Part model, mm, in its own coordinate system. A direction names the side the tool comes from. Round coordinates to 2 decimals unless told otherwise and drop trailing zeros. Loops run counter-clockwise (first coordinate to the right, second up) from the corner with the lowest first, then second, coordinate; pieces in that order, holes last. Notation, with made-up numbers: M 69,3.25 L 74,3.25 A22 ccw 74,22.25 Z; hole C 78.5,36 d5. An arc over 180 degrees is marked long. Write each question's results on one line, items separated by ' | '.
Autodesk Inventor part; units mm, degrees
ref_plane "YZ Plane" through (0, 0, 0) normal (1, 0, 0) x (0, 1, 0)
ref_plane "XZ Plane" through (0, 0, 0) normal (0, 1, 0) x (-1, 0, 0)
ref_plane "XY Plane" through (0, 0, 0) normal (0, 0, 1) x (1, 0, 0)
sketch "Sketch1" plane through (0, 0, 0) normal (0, 1, 0) x (-1, 0, 0)
  line L0 (0, 25.4) -> (25.4, 25.4)
  line L1 (25.4, 25.4) -> (25.4, 0)
  line L2 (25.4, 0) -> (0, 0)
  line L3 (0, 0) -> (0, 25.4)
  line L4 (22.225, 22.225) -> (3.175, 22.225)
  line L5 (3.175, 22.225) -> (3.175, 3.175)
  line L6 (3.175, 3.175) -> (22.225, 3.175)
  line L7 (22.225, 3.175) -> (22.225, 22.225)
  dimension "d0" = 25.4
  dimension "d1" = 25.4
  dimension "d2" = 3.175
extrude "Extrusion1" add sketch "Sketch1" along normal blind 609.6
sketch "Sketch2" plane through (-25.4, 0, 25.4) normal (0, 0, 1) x (1, 0, 0)
  circle A0 centre (12.7, 491.5841) radius 3.302
  circle A1 centre (12.7, 452.2611) radius 3.302
  circle A2 centre (12.7, 412.9381) radius 3.302
  circle A3 centre (12.7, 373.6152) radius 3.302
  circle A4 centre (12.7, 334.2922) radius 3.302
  circle A5 centre (12.7, 294.9693) radius 3.302
  circle A6 centre (12.7, 255.6463) radius 3.302
  circle A7 centre (12.7, 216.3233) radius 3.302
  circle A8 centre (12.7, 177.0004) radius 3.302
  circle A9 centre (12.7, 137.6774) radius 3.302
  circle A10 centre (12.7, 98.3544) radius 3.302
  circle A11 centre (12.7, 118.0159) radius 3.302
  circle A12 centre (12.7, 157.3389) radius 3.302
  circle A13 centre (12.7, 196.6619) radius 3.302
  circle A14 centre (12.7, 235.9848) radius 3.302
  circle A15 centre (12.7, 275.3078) radius 3.302
  circle A16 centre (12.7, 314.6307) radius 3.302
  circle A17 centre (12.7, 353.9537) radius 3.302
  circle A18 centre (12.7, 393.2767) radius 3.302
  circle A19 centre (12.7, 432.5996) radius 3.302
  circle A20 centre (12.7, 471.9226) radius 3.302
  circle A21 centre (12.7, 511.2456) radius 3.302
  line L0 (0, 25.4) -> (25.4, 25.4)
  line L1 (0, 25.4) -> (0, 584.2)
  line L2 (25.4, 584.2) -> (0, 584.2)
  line L3 (25.4, 25.4) -> (25.4, 584.2)
extrude "Extrusion2" [suppressed]
sketch "Sketch3" plane through (-25.4, 0, 0) normal (-1, 0, 0) x (0, 0, 1)
  line L0 (25.4, 0) -> (25.4, 609.6)
  line L1 (0, 0) -> (0, 609.6)
  line L2 (0, 511.2456) -> (25.4, 511.2456) construction
  line L3 (0, 373.6152) -> (25.4, 373.6152) construction
  line L4 (0, 235.9848) -> (25.4, 235.9848) construction
  line L5 (0, 98.3544) -> (25.4, 98.3544) construction
  line L6 (12.7, 523.9456) -> (12.7, 479.4956) construction
  line L7 (12.7, 403.7777) -> (12.7, 343.4527) construction
  line L8 (12.7, 258.2098) -> (12.7, 213.7598) construction
  line L9 (12.7, 130.1044) -> (12.7, 85.6544) construction
  circle A0 centre (12.7, 523.9456) radius 3.302
  circle A1 centre (12.7, 479.4956) radius 3.302
  circle A2 centre (12.7, 403.7777) radius 3.302
  circle A3 centre (12.7, 343.4527) radius 3.302
  circle A4 centre (12.7, 258.2098) radius 3.302
  circle A5 centre (12.7, 213.7598) radius 3.302
  circle A6 centre (12.7, 130.1044) radius 3.302
  circle A7 centre (12.7, 85.6544) radius 3.302
  line L10 (0, 304.8) -> (25.4, 304.8) construction
  line L11 (12.7, 334.9625) -> (12.7, 274.6375) construction
  circle A8 centre (12.7, 334.9625) radius 3.302
  circle A9 centre (12.7, 274.6375) radius 3.302
  line L12 (0, 609.6) -> (25.4, 609.6)
  line L13 (0, 107.8794) -> (25.4, 107.8794) construction
  line L14 (25.4, 0) -> (0, 0)
  circle A10 centre (12.7, 596.9) radius 3.302
  circle A11 centre (12.7, 574.675) radius 3.302
  circle A12 centre (12.7, 558.8) radius 3.302
  line L15 (0, 501.7206) -> (25.4, 501.7206) construction
  circle A13 centre (12.7, 12.7) radius 3.302
  circle A14 centre (12.7, 34.925) radius 3.302
  circle A15 centre (12.7, 50.8) radius 3.302
  point P0 (12.7, 235.9848)
  point P1 (12.7, 373.6152)
  point P2 (12.7, 304.8)
  point P3 (12.7, 107.8794)
  point P4 (12.7, 501.7206)
  dimension "d7" = 44.45
  dimension "d8" = 60.325
  dimension "d9" = 44.45
  dimension "d10" = 44.45
  dimension "d11" = 6.604
  dimension "d12" = 6.604
  dimension "d13" = 6.604
  dimension "d14" = 6.604
  dimension "d15" = 6.604
  dimension "d16" = 6.604
  dimension "d17" = 6.604
  dimension "d18" = 6.604
  dimension "d21" = 60.325
  dimension "d22" = 6.604
  dimension "d23" = 6.604
  dimension "d27" = 9.525
  dimension "d28" = 9.525
  dimension "d29" = 98.3544
  dimension "d30" = 235.9848
  dimension "d31" = 235.9848
  dimension "d32" = 98.3544
extrude "Extrusion3" cut sketch "Sketch3" against normal blind 25.4 contours A0 | A1 | A6 | A7 | A8 | A9 | A10 | A11 | A12 | A13 | A14 | A15
sketch "Sketch4" plane through (0, 0, 25.4) normal (1, 0, 0) x (0, 0, -1)
  line L0 (25.4, 0) -> (25.4, 609.6)
  line L1 (0, 0) -> (0, 609.6)
  line L2 (0, 304.8) -> (25.4, 304.8) construction
  line L3 (12.7, 349.25) -> (12.7, 260.35) construction
  circle A0 centre (12.7, 349.25) radius 3.302
  circle A1 centre (12.7, 260.35) radius 3.302
  circle A2 centre (12.7, 368.3) radius 3.302
  circle A3 centre (12.7, 387.35) radius 3.302
  circle A4 centre (12.7, 406.4) radius 3.302
  circle A5 centre (12.7, 425.45) radius 3.302
  circle A6 centre (12.7, 444.5) radius 3.302
  circle A7 centre (12.7, 241.3) radius 3.302
  circle A8 centre (12.7, 222.25) radius 3.302
  circle A9 centre (12.7, 203.2) radius 3.302
  circle A10 centre (12.7, 184.15) radius 3.302
  circle A11 centre (12.7, 165.1) radius 3.302
  point P0 (12.7, 304.8)
  dimension "d33" = 88.9
  dimension "d34" = 6.604
  dimension "d37" = 19.05
  dimension "d44" = 19.05
extrude "Extrusion4" cut sketch "Sketch4" against normal blind 25.4 contours A2 | A3 | A4 | A5 | A6 | A7 | A8 | A9 | A10 | A11
equation "\"d9\" = d7"
equation "\"d10\" = d7"
equation "\"d12\" = d11"
equation "\"d13\" = d11"
equation "\"d14\" = d11"
equation "\"d15\" = d11"
equation "\"d16\" = d11"
equation "\"d17\" = d11"
equation "\"d18\" = d11"
equation "\"d21\" = d8"
equation "\"d22\" = d11"
equation "\"d23\" = d11"
equation "\"d27\" = d28"
properties part number "Chassis V1.500 Part1" material "Aluminum 6061"
Item 1: Drop a flat-ended pin along its axis: P1, Ø4, axis at y = 425.45, z = 12.7, coming from the +X side. Give the stop position or say it passes through.
Filled sheet:
P1: through
Item 2: Two-plate mould, pull along Z, no slides. Class faces 1 (the flat face through (-13, 301, 0)), 2 (the flat face through (-24, 0, 13)), 3 (the flat face through (-13, 301, 3.175)): +Z half, -Z half, draft (parallel to the pull), parting line (faces both ways), or undercut.
Filled sheet:
face 1: -Z half | face 2: draft | face 3: undercut
Item 3: Band-saw the part on B-B on y = 506. Give the cut face in (x, z) (3 decimals), and give its area (3 significant figures).
Filled sheet:
outline: M -25.4,0 L 0,0 L 0,25.4 L -25.4,25.4 Z; hole M -22.225,3.175 L -3.175,3.175 L -3.175,22.225 L -22.225,22.225 Z | area: 282 mm^2
Item 4: Band-saw the part on A-A on x = -14.5. Give the cut face in (y, z) (3 decimals), and give its area (3 significant figures).
Filled sheet:
outline: M 0,0 L 609.6,0 L 609.6,3.175 L 0,3.175 Z; M 0,22.225 L 609.6,22.225 L 609.6,25.4 L 0,25.4 Z | area: 3,870 mm^2
Item 5: Wall check: L1, parallel to X at y = 480, z = 20.75 (3 decimals); L2, parallel to Z at x = -6.75, y = 32.5 (3 decimals); L3, parallel to Z at x = -1.4, y = 387.35. Give the ranges that are in metal, low to high.
Filled sheet:
L1: -25.4 to -22.225, -3.175 to 0 | L2: 0 to 3.175, 22.225 to 25.4 | L3: 0 to 9.4, 16 to 25.4
Item 6: Which spindle directions (+Z, -Z, +X, -X, +Y, -Y) get a long thin tool onto all of the face, cutting with end or side? Do faces 4 (the flat face through (-13, 301, 25.4)), 5 (the flat face through (-13, 301, 22.225)). Say none if no direction does.
Filled sheet:
face 4: +Z, +X, -X, +Y, -Y | face 5: +Y, -Y
